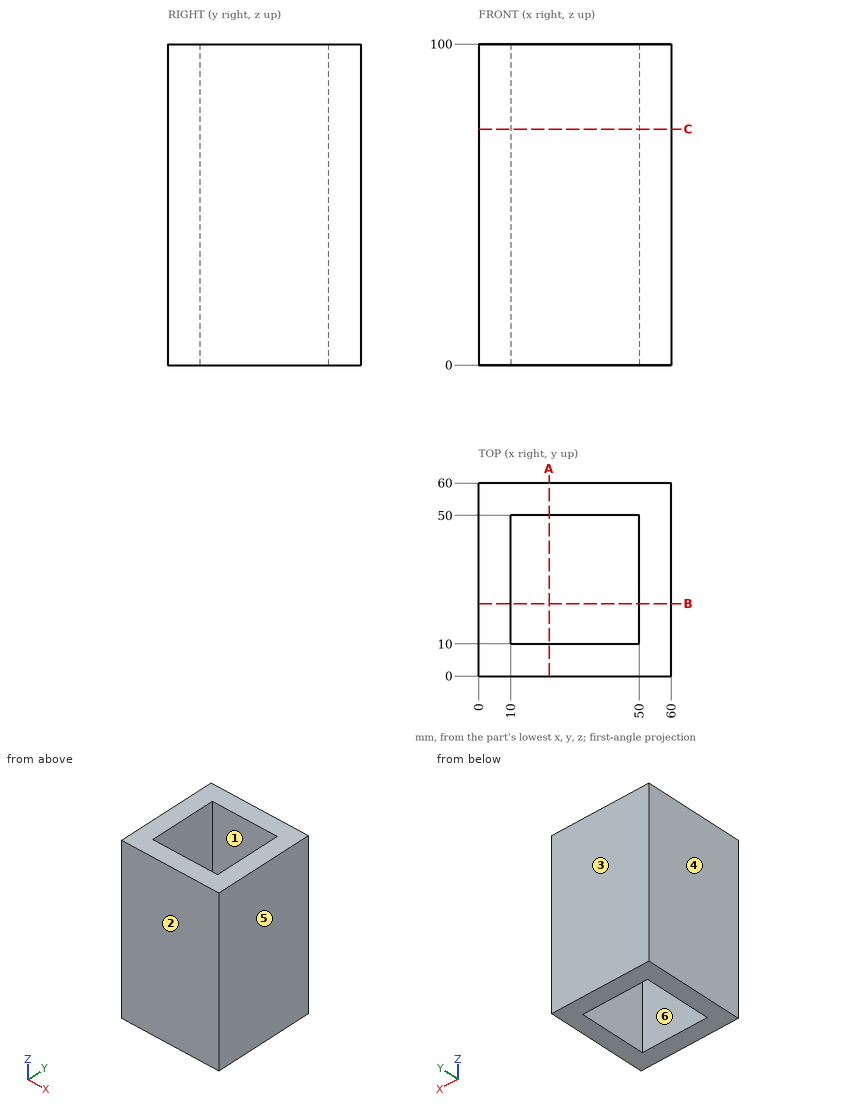
Geometry: see drawing. Coordinates: mm, zero at the bounding-box minimum. A direction names the side the tool comes from. Give positions to 0.01 mm unless a question says otherwise; leave off trailing zeros. Loops run counter-clockwise (first coordinate to the right, second up) from the corner with the lowest first, then second, coordinate; pieces in that order, holes last. Notation, with made-up numbers: (-3, 73.5) - (46, 73.5) arc R19 ccw to (46, 103.5) - close; hole circle Ø9 at (-11.75, 7.25). An arc over 180 degrees is marked (long way). Use CSV: the item, a comma, the result in double quotes. Start each with the question number.
1. Reachability of the marked faces 1 and 2 from +Z, -Z, +X, -X, +Y, -Y: full face, straight path, thin tool, end or side. Return the list, or none.
2. Section A-A (x = 22). Output: boundary loops of the cut face in (y, z), then the cut area to 3 significant figures.
3. Section C-C (z = 73.5). Output: boundary loops of the cut face in (x, y).
4. Ray query, L1, parallel to Y at x = 30, z = 16. Return the intervals inside material, ascending.
5. Draft query along X for the marked faces 3, 4, 5 and 6. Return one class per face: +X half, -X half, draft (parallel to the pull), parting line (faces both ways), or undercut.
Response:
1,face 1,"+Z, -Z"
1,face 2,"+Z, -Z, +X, -X, -Y"
2,outline,"(0, 0) - (10, 0) - (10, 100) - (0, 100) - close; (50, 0) - (60, 0) - (60, 100) - (50, 100) - close"
2,area,"2,000 mm²"
3,outline,"(0, 0) - (60, 0) - (60, 60) - (0, 60) - close; hole (10, 10) - (50, 10) - (50, 50) - (10, 50) - close"
4,L1,"0 to 10, 50 to 60"
5,face 3,"draft"
5,face 4,"-X half"
5,face 5,"+X half"
5,face 6,"undercut"
